For this review, take the finished solid that the model builds, in its own axes (mm). A direction names the side the tool comes from. Coordinates: 2 decimals unless noted, no trailing zeros. Loops run counter-clockwise (first coordinate to the right, second up) from the corner with the lowest first, then second, coordinate; pieces in that order, holes last. Notation, with made-up numbers: (47, 10) - (73, 10) arc R23 cw to (73, 21) - close; hole circle Ø3 at (61, 21). An arc over 180 degrees is marked (long way). Answer as a JSON object with one key per item and string values. Group by question number.
Item 1: Clearance check with flat-ended pins moving along their axes: pin 1 (1.5 mm diameter, centred on x = -29.5, z = -26, fed in from -Y); pin 2 (1 mm diameter, centred on x = -32.5, y = 48, fed in from -Z); pin 3 (2.5 mm diameter, centred on x = -6, z = 1.5, fed in from -Y); pin 4 (15 mm diameter, centred on y = 0, z = 0, fed in from +X). State where each tip first meets the part, or that it passes through.
Item 2: Tool access review of faces 1 (the cylindrical face through (3.81, 1.32, -29.97)), 2 (the flat face through (-18.842, -13, 0)), 3 (the flat face through (-2, 16.5, 0)): name each direction out of +Z, -Z, +X, -X, +Y, -Y from which nothing blocks a thin tool from reaching the whole face with its end or side.
Item 3: We need section A-A (z = 0). Give the boundary of the cut face in (x, y).
Item 4: We need section B-B (y = 0). Give the boundary of the cut face in (x, z).
Item 5: To check wall thickness, follow line 1 (X direction, y = 73.5, z = 26); line 2 (X direction, y = 36.5, z = -71); line 3 (Y direction, x = -42, z = -13). State the ranges of each line that lie inside material, in increasing order.
Item 6: We need section C-C (x = -5). Give the boundary of the cut face in (y, z).
Item 7: We need section D-D (x = -46). Give the boundary of the cut face in (y, z).
Item 8: Mouldability with a two-part tool opening along Z and no side actions: class faces 4 (the flat face through (-2, 14, -4)), 5 (the conical face through (-9.27, -32.16, -7.14)), 6 (the flat face through (16.158, -13, 0)) as released by +Z, released by -Z, zero draft, split by the parting line, or undercut.
from build123d import *

# Parameters (mm, degrees)
F3_D     = 25
F2_W     = 8
F2_H     = 8
F4_DEPTH = 50


with BuildPart() as f1:
    # F0 (on Front) → F1 (revolve)
    with BuildSketch(Plane.XZ):
        with BuildLine():
            Line((16.157746, 30), (-8.200476, 30))
            Line((-8.200476, 30), (-25.330789, 77.065149))
            ThreePointArc((-25.330789, 77.065149), (-47.645877, 86.518166), (-32.521118, 67.582371))
            Line((-32.521118, 67.582371), (-18.842254, 30))
            Line((-18.842254, 30), (-18.842254, 0))
            Line((-18.842254, 0), (16.157746, 0))
            Line((16.157746, 0), (16.157746, 30))
        make_face()
    revolve(axis=Axis((-63.210286, 0, 0), (-1, 0, 0)))

    # F3 (through all)
    with Locations(Plane(origin=(-18.842254, 0, 0), x_dir=(0, -1, 0), z_dir=(-1, 0, 0))):
        with Locations((0, 0)):
            Hole(F3_D / 2)

    # F2 (on face) → F4 (cut)
    with BuildSketch(Plane(origin=(-18.842254, 0, 0), x_dir=(0, -1, 0), z_dir=(-1, 0, 0))):
        with Locations((-12.5, 0)):
            Rectangle(F2_W, F2_H)
    extrude(amount=-F4_DEPTH, mode=Mode.SUBTRACT)


solid = f1.part
Check sheet entries:
{
 "1": {"pin 1": "stops at y = -85.17", "pin 2": "stops at z = -76.94", "pin 3": "stops at y = -30", "pin 4": "passes through"},
 "2": {"face 1": "+X", "face 2": "-X", "face 3": "+X, -X"},
 "3": {"outline": "(-32.52, -67.58) arc R12.5 ccw (long way) to (-25.33, -77.07) - (-8.2, -30) - (16.16, -30) - (16.16, -12.5) - (-18.84, -12.5) - (-18.84, -30) - close; (-32.52, 67.58) - (-18.84, 30) - (-18.84, 16.5) - (16.16, 16.5) - (16.16, 30) - (-8.2, 30) - (-25.33, 77.07) arc R12.5 ccw (long way) to start"},
 "4": {"outline": "(-32.52, -67.58) arc R12.5 ccw (long way) to (-25.33, -77.07) - (-8.2, -30) - (16.16, -30) - (16.16, -12.5) - (-18.84, -12.5) - (-18.84, -30) - close; (-32.52, 67.58) - (-18.84, 30) - (-18.84, 12.5) - (16.16, 12.5) - (16.16, 30) - (-8.2, 30) - (-25.33, 77.07) arc R12.5 ccw (long way) to start"},
 "5": {"line 1": "x = -50.15 to -25.23", "line 2": "x = -50.16 to -25.22", "line 3": "y = -89.76 to -65.97, 65.97 to 89.76"},
 "6": {"outline": "circle Ø60 at (0, 0); hole (11.84, -4) - (16.5, -4) - (16.5, 4) - (11.84, 4) arc R12.5 ccw (long way) to start"},
 "7": {"outline": "circle Ø176.6 at (0, 0); hole circle Ø139.26 at (0, 0)"},
 "8": {"face 4": "undercut", "face 5": "split by the parting line", "face 6": "zero draft"}
}
